Check sheet for the modelled part. Datum: model origin and axes. Units: mm. A direction names the side the tool comes from. Coordinates: 2 decimals unless noted, no trailing zeros. Loops run counter-clockwise (first coordinate to the right, second up) from the corner with the lowest first, then second, coordinate; pieces in that order, holes last. Notation, with made-up numbers: (-18.75, -16.5) -> (40.25, -16.5) arc R23 cw to (40.25, 1.5) -> close; hole circle Ø9 at (-33.5, 36.25). An arc over 180 degrees is marked (long way). Use CSV: the item, a comma, the result in double quotes.
```python
from build123d import *

# Parameters (mm, degrees)
CHAMFER1_SIZE      = 0.6
CUT_EXTRUDE1_DEPTH = 3


with BuildPart() as part:
    # Sketch1 → Revolve1 (revolve)
    with BuildSketch(Plane.XY):
        Polygon((-6, 0), (-6, 4.4), (-5.4, 5), (0, 5), (0, 3), (16, 3), (16, 0), align=None)
    revolve(axis=Axis((16, 0, 0), (-1, 0, 0)))

    # Chamfer1
    chamfer1_edges = [part.edges().sort_by_distance(p)[0] for p in [
        (16, -3, 0),
    ]]
    chamfer(chamfer1_edges, length=CHAMFER1_SIZE)

    # Sketch2 → Cut-Revolve1 (revolve, cut)
    with BuildSketch(Plane.XY):
        Polygon((-6, 0), (-6, 2.5), (-3, 2.5), (-2.330127019, 0), align=None)
    revolve(axis=Axis((-2.330127019, 0, 0), (-1, 0, 0)), mode=Mode.SUBTRACT)

    # Sketch3 → Cut-Extrude1 (cut)
    with BuildSketch(Plane(origin=(-6, 0, 0), x_dir=(0, 0, -1), z_dir=(1, 0, 0))):
        Polygon((-2.5, 1.443375673), (-2.5, -1.443375673), (0, -2.886751346), (2.5, -1.443375673), (2.5, 1.443375673), (0, 2.886751346), align=None)
    extrude(amount=CUT_EXTRUDE1_DEPTH, mode=Mode.SUBTRACT)


solid = part.part
```
1) Go/stop test with flat-tipped pins: pin 1 Ø1.4 at (y, z) = (-1, 2) entering from -X; pin 2 Ø5 at (x, y) = (9.5, 0) entering from +Z; pin 3 Ø2 at (x, z) = (-1.5, 3.5) entering from +Y; pin 4 Ø1 at (x, z) = (4, 2) entering from +Y. Record where each tip stops, or that it passes through.
Answer below:
pin 1,"stops at x = -6"
pin 2,"stops at z = 3"
pin 3,"stops at y = 4.33"
pin 4,"stops at y = 2.6"
2) Draft check along Y on faces 4 (the cylindrical face through (8, -3, 0)), 5 (the conical face through (-2.363, -0.096, 0.074)), 6 (the flat face through (16, 0, 0)). Enter one of: released by +Y, released by -Y, zero draft, split by the parting line, or undercut.
Answer below:
face 4,"split by the parting line"
face 5,"undercut"
face 6,"zero draft"
3) Access from +Z, -Z, +X, -X, +Y, -Y to the whole of each face (thin tool, end or side, straight path). Record for faces 1 (the flat face through (-4.521, -2.175, -1.233)), 2 (the flat face through (0, 3.3, -0.1)), 3 (the flat face through (-6, -2, 2)).
Answer below:
face 1,"-X"
face 2,"+X"
face 3,"+Z, -Z, -X, +Y, -Y"
4) Cross-section at B-B on x = -0.75. Record the boundary of the cut face in (y, z), and give its area (3 significant figures).
Answer below:
outline,"circle Ø10 at (0, 0)"
area,"78.5 mm²"
5) Thickness scan on line 1 along X through (y, z) = (3.25, -2.75); line 2 along Z through (x, y) = (-3.25, -0.5); line 3 along Y through (x, z) = (10, 0.75). Record the ranges inside material, lowest first. Write a range as from..to.
Answer below:
line 1,"x = -6..0"
line 2,"z = -4.97..-2.5, 2.5..4.97"
line 3,"y = -2.9..2.9"
6) Cross-section at C-C on x = 10.75. Record the boundary of the cut face in (y, z), and give its area (3 significant figures).
Answer below:
outline,"circle Ø6 at (0, 0)"
area,"28.3 mm²"
7) Cross-section at A-A on x = -3.25. Record the boundary of the cut face in (y, z), and give its area (3 significant figures).
Answer below:
outline,"circle Ø10 at (0, 0); hole (-2.89, 0) -> (-1.44, -2.5) -> (1.44, -2.5) -> (2.89, 0) -> (1.44, 2.5) -> (-1.44, 2.5) -> close"
area,"56.9 mm²"
